```python
from build123d import *

# Parameters (mm, degrees)
F2_R = 6


with BuildPart() as f1:
    # F0 (on Right) → F1 (revolve)
    with BuildSketch(Plane.YZ):
        with BuildLine():
            Line((0, 31), (-44, 31))
            Line((-44, 31), (-44, 0))
            Line((-44, 0), (24, 0))
            Line((24, 0), (24, 31))
            Line((24, 31), (12, 31))
            ThreePointArc((12, 31), (6, 25), (0, 31))
        make_face()
    revolve(axis=Axis((0, 4.568492, 0), (0, 1, 0)))

    # F2
    f2_edges = [f1.edges().sort_by_distance(p)[0] for p in [
        (0, -44, -31),
    ]]
    fillet(f2_edges, radius=F2_R)

    # F3 (on Right) → F4 (revolve)
    with BuildSketch(Plane.YZ):
        Polygon((41, 20), (24, 20), (24, 0), (44, 0), (44, 16), (41, 16), align=None)
    revolve(axis=Axis((0, 39.701345, 0), (0, 1, 0)))

    # F5 (on Right) → F6 (revolve, cut)
    with BuildSketch(Plane.YZ):
        Polygon((-42.5, 25), (-44, 25), (-44, 0), (44, 0), (44, 6), (-14, 6), (-14, 16), (-22, 16), (-22, 20.5), (-29, 20.5), (-29, 12.5), (-32, 12.5), (-32, 16), (-42.5, 16), align=None)
    revolve(axis=Axis((0, 2.262007, 0), (0, 1, 0)), mode=Mode.SUBTRACT)


solid = f1.part
```
The model under review builds one solid part; all positions refer to its coordinate system, in mm. A direction names the side the tool comes from. Round coordinates to 2 decimals unless told otherwise and drop trailing zeros. Order: outer loops, then holes, each group sorted by start corner. A loop starts at its lowest first (then second) coordinate and runs counter-clockwise, first axis right, second up. Notation, with made-up numbers: (52.25, -26) - (90.25, -26) arc R23 cw to (90.25, 0) - close; hole circle Ø3 at (-34, 11). An arc over 180 degrees is marked (long way). Answer in a Markdown table with one row per item.
(1) Machinability: for faces 1 (the face through (-15.62, 42.48, -3.47)), 2 (the face through (-15.62, -37.32, -3.47)), 3 (the face through (-9, -29, -9)), 4 (the face through (0, 15, -6)), which of the approach directions +Z, -Z, +X, -X, +Y, -Y give a long, thin tool a straight path to every point of the face, cutting with its end or side? Answer none if there is none.
Result set:
| item | result |
|---|---|
| face 1 | +Y |
| face 2 | -Y |
| face 3 | none |
| face 4 | +Y, -Y |
(2) Clearance check with flat-ended pins moving along their axes: P1, Ø16, axis at x = -6, z = 4.5, coming from the -Y side; P2, Ø15.5, axis at x = 0, z = 0, coming from the +Y side; P3, Ø25, axis at x = 4.5, z = -6, coming from the -Y side; P4, Ø4, axis at y = -16.5, z = -14.5, coming from the -X side. State where each tip first meets the part, or that it passes through.
Result set:
| item | result |
|---|---|
| P1 | stops at y = -32 |
| P2 | stops at y = 44 |
| P3 | stops at y = -42.5 |
| P4 | stops at x = -28.37 |
(3) Mouldability with a two-part tool opening along X and no side actions: class faces 5 (the face through (30.736, -19.266, -4.036)), 6 (the face through (3.755, -30.521, 11.923)), 7 (the face through (13.43, 41, 8.98)) as released by +X, released by -X, zero draft, split by the parting line, or undercut.
Result set:
| item | result |
|---|---|
| face 5 | split by the parting line |
| face 6 | undercut |
| face 7 | zero draft |
(4) For line 1 (Y direction, x = -18.5, z = -5.5); line 2 (Y direction, x = -5.5, z = 12.5); line 3 (X direction, y = 21.5, z = 0), list the stretches that pass through material, from the lowest coordinate up. Write a range as from..to.
Result set:
| item | result |
|---|---|
| line 1 | y = -42.5..-29, -22..41 |
| line 2 | y = -32..-29, -14..44 |
| line 3 | x = -31..-6, 6..31 |
(5) Take a section at A-A on y = -1.5. Write out the cut boundary in (x, z), plus the area to 3 significant figures.
Result set:
| item | result |
|---|---|
| outline | circle Ø62 at (0, 0); hole circle Ø12 at (0, 0) |
| area | 2,910 mm2 |
(6) Take a section at B-B on y = -27. Write out the cut boundary in (x, z).
Result set:
| item | result |
|---|---|
| outline | circle Ø62 at (0, 0); hole circle Ø41 at (0, 0) |
